from build123d import *

# Parameters (mm, degrees)
F1_DEPTH  = 6.35
F3_D      = 3.6576
F5_DEPTH  = 6.35
F7_DEPTH  = 12.701
F9_DEPTH  = 6.35
F10_R     = 3.81
F11_DEPTH = 3.175


with BuildPart() as f1:
    # F0 (on Top) → F1 (new body)
    with BuildSketch(Plane.XY):
        with BuildLine():
            ThreePointArc((0, 7.62), (2.2318463274, 2.2318463274), (7.62, 0))
            Line((7.62, 0), (36.83, 0))
            ThreePointArc((36.83, 0), (42.2181536726, 2.2318463274), (44.45, 7.62))
            ThreePointArc((44.45, 7.62), (42.2181536726, 13.0081536726), (36.83, 15.24))
            Line((36.83, 15.24), (7.62, 15.24))
            ThreePointArc((7.62, 15.24), (2.2318463274, 13.0081536726), (0, 7.62))
        make_face()
    extrude(amount=F1_DEPTH)

    # F3 (through all)
    with Locations(Plane.XY.offset(6.35)):
        with Locations((7.62, 7.62)):
            Hole(F3_D / 2)

    # F4 (on face) → F5 (join)
    with BuildSketch(Plane.XY.offset(6.35)):
        with BuildLine():
            Line((36.83, 15.24), (25.4, 15.24))
            Line((25.4, 15.24), (25.4, 0))
            Line((25.4, 0), (36.83, 0))
            ThreePointArc((36.83, 0), (44.45, 7.62), (36.83, 15.24))
        make_face()
    extrude(amount=F5_DEPTH)

    # F6 (on face) → F7 (cut, through all)
    with BuildSketch(Plane.XY.offset(12.7)):
        with BuildLine():
            ThreePointArc((31.75, 11.43), (27.94, 7.62), (31.75, 3.81))
            Line((31.75, 3.81), (36.83, 3.81))
            ThreePointArc((36.83, 3.81), (40.64, 7.62), (36.83, 11.43))
            Line((36.83, 11.43), (31.75, 11.43))
        make_face()
    extrude(amount=-F7_DEPTH, mode=Mode.SUBTRACT)

    # F8 (on face) → F9 (cut)
    with BuildSketch(Plane.XY.offset(12.7)):
        with BuildLine():
            ThreePointArc((31.75, 12.7), (26.67, 7.62), (31.75, 2.54))
            Line((31.75, 2.54), (36.83, 2.54))
            ThreePointArc((36.83, 2.54), (41.91, 7.62), (36.83, 12.7))
            Line((36.83, 12.7), (31.75, 12.7))
        make_face()
    extrude(amount=-F9_DEPTH, mode=Mode.SUBTRACT)

    # F10 (on face) → F11 (cut)
    with BuildSketch(Plane(origin=(0, 0, 0), x_dir=(1, 0, 0), z_dir=(0, 0, -1))):
        with Locations((7.62, -7.62)):
            Circle(F10_R)
    extrude(amount=-F11_DEPTH, mode=Mode.SUBTRACT)


solid = f1.part
Geometry: final body of the model. Coordinates: model frame, mm. A direction names the side the tool comes from. Give positions to 0.01 mm unless a question says otherwise; leave off trailing zeros. Write each loop counter-clockwise with the first axis right and the second up, starting at its lowest first coordinate (ties: lowest second). Pieces come first, ordered by that corner, then holes.
(1) Ray query, line 1 (X direction, y = 7.62, z = 1.7); line 2 (Y direction, x = 32.5, z = 3.75); line 3 (X direction, y = 8, z = 3.25). Return the intervals inside material, ascending.
(2) Cut plane C-C, the plane z = 3.75. Return loops of the section in (x, y), then the cut area to 3 significant figures.
(3) Mould query, pull axis Y, two halves, no side actions, for faces 5 (the flat face through (26, 15.24, 5)), 6 (the cylindrical face through (26.67, 7.73, 9.57)), 7 (the flat face through (25, 0, 5)). Classes: released by +Y, released by -Y, zero draft, split by the parting line, or undercut.
(4) Access query for faces 1 (the cylindrical face through (40.64, 7.54, 3.22)), 2 (the flat face through (13, 8, 6.35)), 3 (the cylindrical face through (11.254, 6.476, 1.565)), 4 (the flat face through (34, 2.54, 10)). Directions: +Z, -Z, +X, -X, +Y, -Y. A direction counts if a zero-diameter tool reaches every point of the face in a straight line with its end or side. Return the directions, or none.
(5) Cut plane B-B, the plane y = 4.75. Return loops of the section in (x, z) (3 decimals).
(6) Cut plane D-D, the plane x = 10.5. Return loops of the section in (y, z) (3 decimals).
(7) First-contact query: P1, Ø6, axis at y = 13, z = 4.5, coming from the +X side; P2, Ø2, axis at x = 8, z = 8.5, coming from the -Y side; P3, Ø8.5, axis at x = 6.5, y = 6.5, coming from the -Z side; P4, Ø3, axis at y = 9.5, z = 10.5, coming from the -X side. Flat tips, straight axial feed; report the tip coordinate or a pass-through.
(8) Cut plane A-A, the plane z = 8.25. Return loops of the section in (x, y).
Values follow:
1. line 1: x = 0 to 3.81, 11.43 to 27.94, 40.64 to 44.45
1. line 2: y = 0 to 3.81, 11.43 to 15.24
1. line 3: x = 0.01 to 5.83, 9.41 to 27.96, 40.62 to 44.44
2. outline: (7.62, 0) - (36.83, 0) arc R7.62 ccw to (36.83, 15.24) - (7.62, 15.24) arc R7.62 ccw to start; hole circle Ø3.66 at (7.62, 7.62); hole (31.75, 3.81) - (36.83, 3.81) arc R3.81 ccw to (36.83, 11.43) - (31.75, 11.43) arc R3.81 ccw to start
2. area: 533 mm2
3. face 5: released by +Y
3. face 6: undercut
3. face 7: released by -Y
4. face 1: +Z, -Z
4. face 2: +Z, -X, +Y, -Y
4. face 3: -Z
4. face 4: +Z
5. outline: (0.561, 0) - (5.114, 0) - (5.114, 3.175) - (10.126, 3.175) - (10.126, 0) - (29.244, 0) - (29.244, 6.35) - (27.558, 6.35) - (27.558, 12.7) - (25.4, 12.7) - (25.4, 6.35) - (0.561, 6.35) - close; (39.336, 0) - (43.889, 0) - (43.889, 12.7) - (41.022, 12.7) - (41.022, 6.35) - (39.336, 6.35) - close
6. outline: (0, 0) - (5.126, 0) - (5.126, 3.175) - (10.114, 3.175) - (10.114, 0) - (15.24, 0) - (15.24, 6.35) - (0, 6.35) - close
7. P1: stops at x = 44.07
7. P2: passes through
7. P3: stops at z = 0
7. P4: stops at x = 25.4
8. outline: (25.4, 0) - (36.83, 0) arc R7.62 ccw to (36.83, 15.24) - (25.4, 15.24) - close; hole (31.75, 2.54) - (36.83, 2.54) arc R5.08 ccw to (36.83, 12.7) - (31.75, 12.7) arc R5.08 ccw to start
